Work out the finished part from the listing and answer in its coordinate system (mm). A direction names the side the tool comes from. Round coordinates to 2 decimals unless told otherwise and drop trailing zeros. Order: outer loops, then holes, each group sorted by start corner. A loop starts at its lowest first (then second) coordinate and runs counter-clockwise, first axis right, second up. Notation, with made-up numbers: (19, 71) - (42, 71) arc R16 cw to (42, 87) - close; hole circle Ø5 at (80, 27.25). An arc over 180 degrees is marked (long way). Put each result on its own line as item: value.
```python
from build123d import *

# Parameters (mm, degrees)
BOSS_EXTRUDE1_DEPTH = 2
BOSS_EXTRUDE2_DEPTH = 13.6
CUT_EXTRUDE1_DEPTH  = 204.774312539
TOP_HOLES_D         = 3.2
TOP_HOLES_DEPTH     = 1.2
WRIST_1_D           = 3.2
WRIST_1_DEPTH       = 1.2
WRIST_2_D           = 3.2
WRIST_2_DEPTH       = 1.2
WRIST_3_D           = 3.2
WRIST_3_DEPTH       = 1.2
FILLET1_R           = 5
FILLET2_R           = 10
FILLET3_R           = 10


with BuildPart() as part:
    # outline → Boss-Extrude1 (new body)
    with BuildSketch(Plane(origin=(0, 0, 0), x_dir=(1, 0, 0), z_dir=(0, 1, 0))):
        Polygon((22.752080985, 112.217917805), (22.752080985, 32.585832501), (25.688129691, 26.292829341), (39.910245267, 1.671913524), (75.213887712, 15.680109343), (93.764616437, 15.680109343), (112.21601573, 10.581860359), (131.186066133, 10.581860359), (140.397681326, 25.454275085), (160.788080985, 27.045655036), (160.788080985, 105.9953847), (121.597788595, 112.217917805), align=None)
    extrude(amount=BOSS_EXTRUDE1_DEPTH)

    # outline<7> → Boss-Extrude2 (add)
    with BuildSketch(Plane(origin=(0, 0, 0), x_dir=(1, 0, 0), z_dir=(0, 1, 0))):
        Polygon((165.988080985, 110.434880876), (122.008040315, 117.417917805), (17.552080985, 117.417917805), (17.552080985, 31.432460189), (21.071788866, 23.888466533), (37.653795388, -4.817824349), (76.207852469, 10.480109343), (93.059430407, 10.480109343), (111.510829699, 5.381860359), (134.081949487, 5.381860359), (143.430369308, 20.475150048), (165.988080985, 22.235679058), align=None)
        Polygon((121.597788595, 112.217917805), (22.752080985, 112.217917805), (22.752080985, 32.585832501), (25.688129691, 26.292829341), (39.910245267, 1.671913524), (75.213887712, 15.680109343), (93.764616437, 15.680109343), (112.21601573, 10.581860359), (131.186066133, 10.581860359), (140.397681326, 25.454275085), (160.788080985, 27.045655036), (160.788080985, 105.9953847), align=None, mode=Mode.SUBTRACT)
    extrude(amount=BOSS_EXTRUDE2_DEPTH)

    # cutout → Cut-Extrude1 (cut, through all)
    with BuildSketch(Plane(origin=(0, 0, 0), x_dir=(1, 0, 0), z_dir=(0, 1, 0))):
        Polygon((17.552080985, 117.417917805), (17.552080985, 52.217917805), (22.752080985, 52.217917805), (22.752080985, 112.217917805), (47.752080985, 112.217917805), (47.752080985, 117.417917805), align=None)
    extrude(amount=CUT_EXTRUDE1_DEPTH, mode=Mode.SUBTRACT)

    # top holes
    with Locations(Plane(origin=(0, 13.6, 0), x_dir=(1, 0, 0), z_dir=(0, 1, 0))):
        with Locations((84.67493479, 114.817917805), (20.152080985, 32.009146345), (38.782020327, -1.572955412), (75.710870091, 13.080109343), (111.863422715, 7.981860359), (163.388080985, 24.640667047), (163.388080985, 108.215132788), (121.802914455, 114.817917805)):
            Hole(TOP_HOLES_D / 2, depth=TOP_HOLES_DEPTH)

    # wrist 1
    with Locations(Plane.XY.offset(-10.480109343)):
        with Locations((84.633641438, 6.8)):
            Hole(WRIST_1_D / 2, depth=WRIST_1_DEPTH)

    # wrist 2
    with Locations(Plane.XY.offset(-5.381860359)):
        with Locations((122.796389593, 6.8)):
            Hole(WRIST_2_D / 2, depth=WRIST_2_DEPTH)

    # wrist 3
    with Locations(Plane(origin=(-0.719959147, 0, -9.224858415), x_dir=(0.9969682889311796, 0, -0.07780893821172487), z_dir=(0.07780893821172487, 0, 0.9969682889311796))):
        with Locations((155.901833608, 6.8)):
            Hole(WRIST_3_D / 2, depth=WRIST_3_DEPTH)

    # Fillet1
    fillet1_edges = [part.edges().sort_by_distance(p)[0] for p in [
        (22.752080985, 1, -112.217917805),
    ]]
    fillet(fillet1_edges, radius=FILLET1_R)

    # Fillet2
    # the kernel refuses this fillet: 10 mm, written as the material it takes off along each edge
    with BuildSketch(Plane(origin=(47.752080985, -21.931712199, -117.417917805), x_dir=(0, 0, 1), z_dir=(0, 1, 0))) as fillet2_piece_1:
        with BuildLine():
            CenterArc((10, 8.77268488), FILLET2_R, 180, 61.314597986)
            Line((0, 8.77268488), (-0.2, 8.77268488))
            Line((-0.2, 8.77268488), (-0.2, 0))
            Line((-0.2, 0), (0, -0.2))
            ThreePointArc((0, -0.2), (2.6, -0.2), (5.104, -0.175453698))
            Line((5.104, -0.175453698), (5.2, 0))
        make_face()
    extrude(amount=57.463424399, mode=Mode.SUBTRACT)

    # Fillet3
    # the kernel refuses this fillet: 10 mm, written as the material it takes off along each edge
    with BuildSketch(Plane(origin=(17.552080985, -21.931712199, -52.217917805), x_dir=(0, 0, 1), z_dir=(0, 1, 0))) as fillet3_piece_1:
        with BuildLine():
            CenterArc((8.77268488, 10), FILLET3_R, 208.685402014, 61.314597986)
            Line((0, 5.2), (-0.175453698, 5.104))
            ThreePointArc((-0.175453698, 5.104), (-0.2, 2.6), (-0.2, 0))
            Line((-0.2, 0), (0, -0.2))
            Line((0, -0.2), (8.77268488, -0.2))
            Line((8.77268488, -0.2), (8.77268488, 0))
        make_face()
    extrude(amount=57.463424399, mode=Mode.SUBTRACT)


solid = part.part
```
1) Straight lines are drawn through the part: L1, parallel to Z at x = 113, y = 3; L2, parallel to X at y = 7.5, z = -37; L3, parallel to X at y = 1, z = -90. For each, find the intervals that lie inside material, in ascending order. Write a range as from..to.
Findings below:
L1: z = -117.42..-112.22, -10.58..-5.38
L2: x = 17.55..22.75, 160.79..165.99
L3: x = 22.75..165.99
2) Given pin 1 Ø1.9 at (x, z) = (111.86, -7.98) entering from +Y; pin 2 Ø4 at (y, z) = (10.5, -90.5) entering from -X; pin 3 Ø8 at (x, z) = (149.5, -101.5) entering from +Y, each flat-ended and moving along its own axis, determine where each tip first touches the part or whether it passes through.
Findings below:
pin 1: stops at y = 12.4
pin 2: stops at x = 160.79
pin 3: stops at y = 2
3) For a pull along Y with two mould halves and no side action, classify faces 4 (the flat face through (123, 7, -6.582)), 5 (the flat face through (112, 12.4, -8)), 6 (the flat face through (85, 5, -10.48)) as pulls with the +Y half, pulls with the -Y half, needs draft (parallel to the pull), parting line crosses it, or undercut.
Findings below:
face 4: undercut
face 5: pulls with the +Y half
face 6: needs draft
4) For faces 1 (the cylindrical face through (37.256, 12.992, 1.092)), 2 (the flat face through (19.29, 6.7, -27.71)), 3 (the flat face through (85, 8, -112.218)), determine the directions among +Z, -Z, +X, -X, +Y, -Y from which every point of the face is accessible in a straight line to the end or side of a thin tool.
Findings below:
face 1: +Y
face 2: +Z, -X, +Y, -Y
face 3: -X, +Y
5) A cutting plane is placed at C-C on x = 67. Write down the section's boundary in (y, z).
Findings below:
outline: (0, -117.42) - (13.6, -117.42) - (13.6, -112.22) - (2, -112.22) - (2, -12.42) - (13.6, -12.42) - (13.6, -6.83) - (0, -6.83) - close
6) A cutting plane is placed at A-A on z = -64. Write down the section's boundary in (x, y).
Findings below:
outline: (22.75, 0) - (165.99, 0) - (165.99, 13.6) - (160.79, 13.6) - (160.79, 2) - (22.75, 2) - close
7) A cutting plane is placed at B-B on x = 106. Write down the section's boundary in (y, z).
Findings below:
outline: (0, -117.42) - (13.6, -117.42) - (13.6, -112.22) - (2, -112.22) - (2, -12.3) - (13.6, -12.3) - (13.6, -6.9) - (0, -6.9) - close
